Input: part model. Units: mm. Frame: model coordinates. A direction names the side the tool comes from. Give positions to 0.01 mm unless a question says otherwise; leave off trailing zeros. Order: outer loops, then holes, each group sorted by start corner. A loop starts at its lowest first (then second) coordinate and runs counter-clockwise, first axis right, second up. Notation, with made-up numbers: M 52,15.5 L 97,15.5 A8 cw 97,22.5 Z; hole C 75.25,75.25 d3. An arc over 180 degrees is marked long. Use a Markdown table: item, result.
from build123d import *

# Parameters (mm, degrees)
SKETCH1_W          = 115
SKETCH1_H          = 115
BASE_DEPTH         = 5
SKETCH2_W          = 115
SKETCH2_H          = 15
SKETCH2_W_2        = 105
SKETCH2_H_2        = 5.16
FRAME1_DEPTH       = 5
FRAME2_START       = -5
FRAME2_DEPTH       = 5
SKETCH5_W          = 5
SKETCH5_H          = 5
POST_DEPTH         = 15
SKETCH6_W          = 1.746666666
SKETCH6_H          = 105
SKETCH6_W_2        = 105
SKETCH6_H_2        = 1.746666666
TRACKS_DEPTH       = 1.666666667
CUT_EXTRUDE1_DEPTH = 1.67


with BuildPart() as part:
    # Sketch1 → Base (new body)
    with BuildSketch(Plane(origin=(0, 0, 0), x_dir=(1, 0, 0), z_dir=(0, 1, 0))):
        Rectangle(SKETCH1_W, SKETCH1_H)
    extrude(amount=BASE_DEPTH)

    # Sketch2 → Frame1 (add)
    with BuildSketch(Plane.ZY.offset(57.5)):
        with Locations((0, 12.5)):
            Rectangle(SKETCH2_W, SKETCH2_H)
        with Locations((0, 12.5)):
            Rectangle(SKETCH2_W_2, SKETCH2_H_2, mode=Mode.SUBTRACT)
    extrude(amount=-FRAME1_DEPTH)

    # Sketch4 → Frame2 (add)
    with BuildSketch(Plane(origin=(0, 0, -57.5), x_dir=(-1, 0, 0), z_dir=(0, 0, -1)).offset(FRAME2_START)):
        Polygon((-57.5, 5), (-52.5, 5), (-52.5, 10.08), (52.5, 10.08), (52.5, 5), (57.5, 5), (57.5, 20), (52.5, 20), (52.5, 14.92), (-52.5, 14.92), (-52.5, 20), (-57.5, 20), align=None)
    extrude(amount=FRAME2_DEPTH)

    # Sketch5 → Post (add)
    with BuildSketch(Plane(origin=(0, 5, 0), x_dir=(1, 0, 0), z_dir=(0, 1, 0))):
        with Locations((55, -55)):
            Rectangle(SKETCH5_W, SKETCH5_H)
    extrude(amount=POST_DEPTH)

    # Sketch6 → Tracks (cut)
    with BuildSketch(Plane(origin=(0, 5, 0), x_dir=(1, 0, 0), z_dir=(0, 1, 0))):
        with Locations((55, 0)):
            Rectangle(SKETCH6_W, SKETCH6_H)
        with Locations((0, -55)):
            Rectangle(SKETCH6_W_2, SKETCH6_H_2)
    extrude(amount=-TRACKS_DEPTH, mode=Mode.SUBTRACT)

    # Sketch7 → Cut-Extrude1 (cut)
    with BuildSketch(Plane(origin=(0, 5, 0), x_dir=(1, 0, 0), z_dir=(0, 1, 0))):
        Polygon((53.735079844, -52.5), (-51.264920156, 52.5), (-52.5, 52.5), (-52.5, 51.264920156), (52.5, -53.735079844), (52.5, -52.5), align=None)
    extrude(amount=-CUT_EXTRUDE1_DEPTH, mode=Mode.SUBTRACT)


solid = part.part
1) Cut plane C-C on x = -6. Return loops of the section in (y, z), and give its area (3 significant figures).
Response values:
| item | result |
|---|---|
| outline | M 0,-57.5 L 5,-57.5 L 5,-7.24 L 3.33,-7.24 L 3.33,-4.76 L 5,-4.76 L 5,54.13 L 3.33,54.13 L 3.33,55.87 L 5,55.87 L 5,57.5 L 0,57.5 Z; M 10.08,-57.5 L 14.92,-57.5 L 14.92,-52.5 L 10.08,-52.5 Z |
| area | 592 mm² |
2) Cut plane A-A on y = 7.75. Return loops of the section in (x, z), and give its area (3 significant figures).
Response values:
| item | result |
|---|---|
| outline | M -57.5,-57.5 L -52.5,-57.5 L -52.5,57.5 L -57.5,57.5 Z; M 52.5,-57.5 L 57.5,-57.5 L 57.5,-52.5 L 52.5,-52.5 Z; M 52.5,52.5 L 57.5,52.5 L 57.5,57.5 L 52.5,57.5 Z |
| area | 625 mm² |
3) Mould query, pull axis Z, two halves, no side actions, for faces 1 (the face through (57.5, 4, 0)), 2 (the face through (0, 3.33, 0)), 3 (the face through (1, 12, -57.5)). Classes: released by +Z, released by -Z, zero draft, split by the parting line, or undercut.
Response values:
| item | result |
|---|---|
| face 1 | zero draft |
| face 2 | undercut |
| face 3 | released by -Z |
4) First-contact query: pin 1 Ø10 at (x, z) = (-43, 36) entering from +Y; pin 2 Ø3 at (x, y) = (29.5, 9.5) entering from +Z; pin 3 Ø0.5 at (x, z) = (7, 55) entering from +Y. Flat tips, straight axial feed; report the tip coordinate or a pass-through.
Response values:
| item | result |
|---|---|
| pin 1 | stops at y = 5 |
| pin 2 | stops at z = -52.5 |
| pin 3 | stops at y = 3.33 |
5) Reachability of faces 4 (the face through (1.97, 4.177, 0.735)), 5 (the face through (-1, 0, -1)), 6 (the face through (1, 10.08, -55)), 7 (the face through (52.5, 17, -55)), 8 (the face through (-55, 9.92, -1)) from +Z, -Z, +X, -X, +Y, -Y: full face, straight path, thin tool, end or side. Return the list, or none.
Response values:
| item | result |
|---|---|
| face 4 | +Y |
| face 5 | +Z, -Z, +X, -X, -Y |
| face 6 | +Z, -Z |
| face 7 | +Z, -Z, +Y |
| face 8 | +X, -X |
6) Material intervals for line 1 (X direction, y = 4.25, z = 0); line 2 (Y direction, x = 49, z = -41); line 3 (Y direction, x = -45, z = -46), sorted ascending. Write a range as from..to.
Response values:
| item | result |
|---|---|
| line 1 | x = -57.5..-1.24, 1.24..54.13, 55.87..57.5 |
| line 2 | y = 0..5 |
| line 3 | y = 0..3.33 |
7) Cut plane B-B on z = -7.5. Return loops of the section in (x, y).
Response values:
| item | result |
|---|---|
| outline | M -57.5,0 L 57.5,0 L 57.5,5 L 55.87,5 L 55.87,3.33 L 54.13,3.33 L 54.13,5 L -6.26,5 L -6.26,3.33 L -8.74,3.33 L -8.74,5 L -52.5,5 L -52.5,9.92 L -57.5,9.92 Z; M -57.5,15.08 L -52.5,15.08 L -52.5,20 L -57.5,20 Z |
